from build123d import *

# Parameters (mm, degrees)
MAIN_DEPTH          = 4
ESQUISSE2_R         = 2.5
BOSS_EXTRUDE1_DEPTH = 1.8


with BuildPart() as part:
    # Esquisse1 → Main (new body)
    with BuildSketch(Plane.XY):
        with BuildLine():
            Line((-4.375785644, 4.25), (-6.426543071, 6.300757427))
            ThreePointArc((-6.426543071, 6.300757427), (-3.48519606, 8.297795395), (0, 9))
            Line((0, 9), (35, 6))
            ThreePointArc((35, 6), (40.994596048, 0.254594236), (35.508729866, -5.978393925))
            Line((35.508729866, -5.978393925), (0, -9))
            ThreePointArc((0, -9), (-3.48519606, -8.297795395), (-6.426543071, -6.300757427))
            Line((-6.426543071, -6.300757427), (-4.375785644, -4.25))
            ThreePointArc((-4.375785644, -4.25), (0, -6.1), (4.375785644, -4.25))
            Line((4.375785644, -4.25), (17.31559729, -2.78215714))
            ThreePointArc((17.31559729, -2.78215714), (19.8, 0), (17.31559729, 2.78215714))
            Line((17.31559729, 2.78215714), (4.375785644, 4.25))
            ThreePointArc((4.375785644, 4.25), (0, 6.1), (-4.375785644, 4.25))
        make_face()
        with BuildLine():
            Line((23.5, 3.25), (35, 3.25))
            ThreePointArc((35, 3.25), (38.25, 0), (35, -3.25))
            Line((35, -3.25), (23.5, -3.25))
            ThreePointArc((23.5, -3.25), (20.25, 0), (23.5, 3.25))
        make_face(mode=Mode.SUBTRACT)
    extrude(amount=MAIN_DEPTH)

    # Esquisse2 → Boss-Extrude1 (add)
    with BuildSketch(Plane(origin=(0, 0, 4), x_dir=(-1, 0, 0), z_dir=(0, 0, -1))):
        with BuildLine():
            Line((0, -9), (-13.008239171, -7.893067292))
            ThreePointArc((-13.008239171, -7.893067292), (-20.250000727, -0.004029611), (-13.008239171, 7.885008071))
            Line((-13.008239171, 7.885008071), (0, 9))
            ThreePointArc((0, 9), (3.48519606, 8.297795395), (6.426543071, 6.300757427))
            Line((6.426543071, 6.300757427), (6.426543071, -6.300757427))
            ThreePointArc((6.426543071, -6.300757427), (3.48519606, -8.297795395), (0, -9))
        make_face()
        Circle(ESQUISSE2_R, mode=Mode.SUBTRACT)
    extrude(amount=BOSS_EXTRUDE1_DEPTH)


solid = part.part
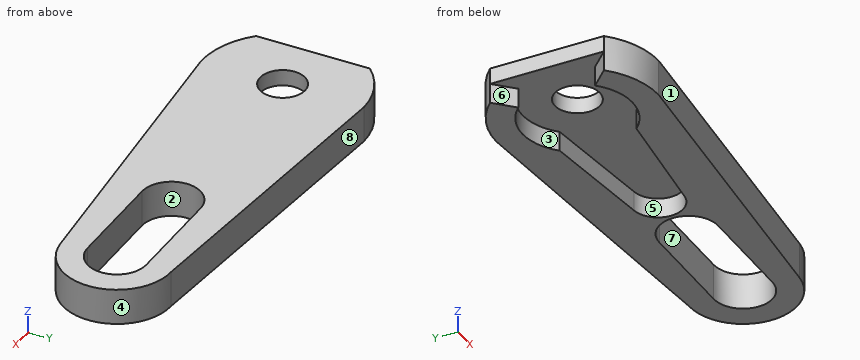
The model under review builds one solid part; all positions refer to its coordinate system, in mm. Face numbers are marked on the shaded views. A direction names the side the tool comes from. Give positions to 0.01 mm unless a question says otherwise; leave off trailing zeros. Write each loop counter-clockwise with the first axis right and the second up, starting at its lowest first coordinate (ties: lowest second). Pieces come first, ordered by that corner, then holes.
1. Add section D-D, the plane x = 3. Write out the cut boundary in (y, z).
2. Add section C-C, the plane y = 5.5. Write out the cut boundary in (x, z).
3. Draft analysis for pull direction X (two halves, no side actions). For the marked faces 6, 7 and 8, state which applies: +X half, -X half, draft (parallel to the pull), parting line (faces both ways), or undercut.
4. Add section A-A, the plane z = 0.75. Write out the cut boundary in (x, y), plus the area to 3 significant figures.
5. Add section B-B, the plane x = 22. Write out the cut boundary in (y, z).
6. Tool access review of the marked faces 1, 2, 3, 4 and 5: name each direction out of +Z, -Z, +X, -X, +Y, -Y from which nothing blocks a thin tool from reaching the whole face with its end or side.
7. For P1, Ø2, axis at x = 31, z = 1.5, coming from the -Y side; P2, Ø4, axis at x = 0, y = 0, coming from the -Z side; P3, Ø6.5, axis at x = 8.5, y = 0, coming from the -Z side; P4, Ø2, axis at x = 18, z = 3, coming from the +Y side, all flat-tipped, find the tip position at first contact; note any pin that passes through.
8. Wall thickness on L1, parallel to Y at x = 0, z = 3; L2, parallel to X at y = 1.75, z = 3.65; L3, parallel to X at y = 1.5, z = 0.7: over which ranges is each line inside the solid? List them lowest first.
Worked answers:
1. outline: (-8.74, 0) - (-5.31, 0) - (-5.31, 2.2) - (5.31, 2.2) - (5.31, 0) - (8.74, 0) - (8.74, 4) - (-8.74, 4) - close
2. outline: (-6.43, 2.2) - (-5.63, 2.2) - (-5.63, 0) - (-2.64, 0) - (-2.64, 2.2) - (2.64, 2.2) - (2.64, 0) - (37.4, 0) - (37.4, 4) - (-6.43, 4) - close
3. face 6: -X half
3. face 7: undercut
3. face 8: +X half
4. outline: (-6.43, -6.3) arc R9 ccw to (0, -9) - (35.51, -5.98) arc R6 ccw to (35, 6) - (0, 9) arc R9 ccw to (-6.43, 6.3) - (-4.38, 4.25) arc R6.1 cw to (4.38, 4.25) - (17.32, 2.78) arc R2.8 cw to (17.32, -2.78) - (4.38, -4.25) arc R6.1 cw to (-4.38, -4.25) - close; hole (23.5, -3.25) - (35, -3.25) arc R3.25 ccw to (35, 3.25) - (23.5, 3.25) arc R3.25 ccw to start
4. area: 359 mm2
5. outline: (-7.13, 0) - (-2.88, 0) - (-2.88, 4) - (-7.13, 4) - close; (2.88, 0) - (7.11, 0) - (7.11, 4) - (2.88, 4) - close
6. face 1: +Z, -Z, +X, -Y
6. face 2: +Z, -Z
6. face 3: -Z
6. face 4: +Z, -Z, +X
6. face 5: -Z, -X
7. P1: stops at y = -6.45
7. P2: passes through
7. P3: stops at z = 2.2
7. P4: stops at y = 7.54
8. L1: y = -9 to -2.5, 2.5 to 9
8. L2: x = -6.43 to -1.79, 1.79 to 20.76, 37.74 to 40.74
8. L3: x = 19.36 to 20.62, 37.88 to 40.81
